For this review, take the finished solid that the model builds, in its own axes (mm). Face numbers are marked on the shaded views. Give positions to 0.01 mm unless a question says otherwise; leave off trailing zeros. Write each loop counter-clockwise with the first axis right and the second up, starting at its lowest first coordinate (ties: lowest second). Pieces come first, ordered by that corner, then holes. Notation, with made-up numbers: M -8,-16.75 L 50,-16.75 A22 ccw 50,19.25 Z; hole C 71,-38 d5. An arc over 180 degrees is marked long. One line per item, written item: value. Start each with the question number.
Item 1: To check wall thickness, follow probe 1 along Y at (x, z) = (0, -4.7); probe 2 along X at (y, z) = (0.5, 4.5); probe 3 along X at (y, z) = (0.5, -4.85). State the ranges of each line that lie inside material, in increasing order.
Item 2: Clearance check with flat-ended pins moving along their axes: pin 1 Ø1.4 at (x, y) = (0, 0.5) entering from +Z; pin 2 Ø2 at (x, y) = (-1, 1.5) entering from -Z. State where each tip first meets the part, or that it passes through.
Item 3: Mouldability with a two-part tool opening along Y and no side actions: class the marked faces 1, 2 and 3 as released by +Y, released by -Y, zero draft, split by the parting line, or undercut.
Item 4: Consider section A-A, the plane y = 4.75. Write out the cut boundary in (x, z), and give its area (3 significant figures).
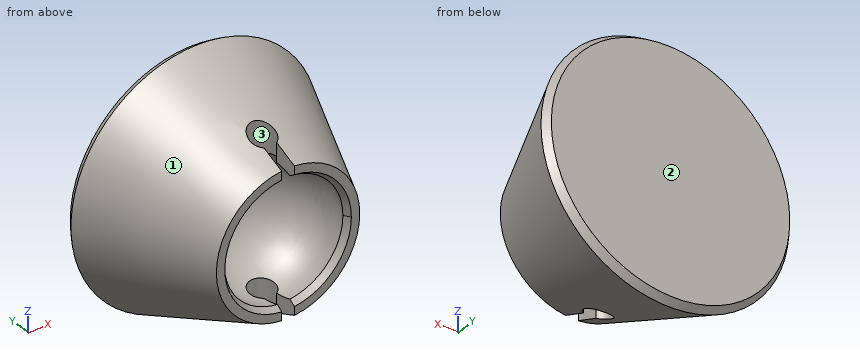
Autodesk Inventor part; units mm, degrees
ref_plane "YZ Plane" through (0, 0, 0) normal (1, 0, 0) x (0, 1, 0)
ref_plane "XZ Plane" through (0, 0, 0) normal (0, 1, 0) x (-1, 0, 0)
ref_plane "XY Plane" through (0, 0, 0) normal (0, 0, 1) x (1, 0, 0)
sketch "Sketch2" plane through (0, 0, 0) normal (0, 0, 1) x (1, 0, 0)
  arc A0 (3.5799, -1.6693) -> (1.25, 3.747) centre (0, 0) ccw
  line L0 (3.5799, -1.6693) -> (4.51, -1.6693)
  line L1 (4.51, -1.6693) -> (7.8046, 6.0923)
  line L2 (7.5, 6.5525) -> (0, 6.5525)
  line L3 (0, 6.5525) -> (0, 4.5525)
  arc A1 (0, 4.5525) -> (1.25, 3.747) centre (2.1994, 6.5928) ccw
  line L4 (0, 0) -> (1.25, 0) construction
  line L5 (7.8046, 6.0923) -> (7.5, 6.5525)
  point P0 (8, 6.5525)
  dimension "d11" = 3.95
  dimension "d12" = 2
  dimension "d13" = 67
  dimension "d14" = 3
  dimension "d15" = 2.5
  dimension "d16" = 25
  dimension "d17" = 0.5
  dimension "d18" = 0.5
  dimension "d19" = 16
  dimension "d20" = 0.9301
revolve "Revolution1" add sketch "Sketch2" angle 360 about axis through (0, 6.5525, 0) along (0, -1, 0)
chamfer "Chamfer1" distance 0.4 angle 45 1 edges at (-3.5799, -1.6693, 0)
sketch "Sketch3" plane through (0, 0, 0) normal (0, 0, 1) x (1, 0, 0)
  arc A0 (3.7304, -1.2987) -> (-3.7304, -1.2987) centre (0, 0) ccw
  line L0 (-3.9799, -1.6693) -> (3.9799, -1.6693)
  line L1 (-0.4, -1.6693) -> (0.4, -1.6693)
  line L2 (0.4, -1.6693) -> (0.4, -0.1928)
  line L3 (0.4, -0.1928) -> (-0.4, -0.1928) construction
  line L4 (-0.4, -0.1928) -> (-0.4, -1.6693)
  line L5 (-0.4, -1.6693) -> (0.4, -0.1928) construction
  line L6 (0.4, -1.6693) -> (-0.4, -0.1928) construction
  arc A1 (0.4, -0.1928) -> (-0.4, -0.1928) centre (0, 0.5) ccw
  point P0 (0, -0.9311)
  dimension "d25" = 0.8
  dimension "d26" = 0.8
  dimension "d27" = 0.5
extrude "Extrusion2" cut sketch "Sketch3" along normal through all both and the other way through all
properties part number "Table Clamp Swiveling Pad" material "SAE 1020"
Model answer:
1. probe 1: y = 1.3 to 6.55
1. probe 2: x = -3.04 to -0.8, 0.8 to 3.04
1. probe 3: x = -2.44 to -0.8, 0.8 to 2.44
2. pin 1: passes through
2. pin 2: stops at z = -6.22
3. face 1: released by -Y
3. face 2: released by +Y
3. face 3: undercut
4. outline: C 0,0 d14.47
4. area: 164 mm2
